from build123d import *

# Parameters (mm, degrees)
SKETCH1_W           = 53
SKETCH1_H           = 16
BOSS_EXTRUDE1_DEPTH = 18
SHELL1_T            = -0.5
SKETCH2_W           = 90
SKETCH2_H           = 20
SKETCH2_R           = 2.5
BOSS_EXTRUDE2_DEPTH = 0.5


with BuildPart() as part:
    # Sketch1 → Boss-Extrude1 (new body)
    with BuildSketch(Plane(origin=(0, 0, 0), x_dir=(0, 0, -1), z_dir=(1, 0, 0))):
        Rectangle(SKETCH1_W, SKETCH1_H)
    extrude(amount=BOSS_EXTRUDE1_DEPTH)

    # Shell1
    shell1_openings = [part.faces().sort_by_distance(p)[0] for p in [
        (18, 0, 0),
    ]]
    offset(amount=SHELL1_T, openings=shell1_openings, kind=Kind.INTERSECTION)

    # Sketch2 → Boss-Extrude2 (add)
    with BuildSketch(Plane(origin=(18, 0, 0), x_dir=(0, 0, -1), z_dir=(1, 0, 0))):
        Rectangle(SKETCH2_W, SKETCH2_H)
        with Locations((36.5, 0)):
            Circle(SKETCH2_R, mode=Mode.SUBTRACT)
        with Locations((-36.5, 0)):
            Circle(SKETCH2_R, mode=Mode.SUBTRACT)
        Polygon((-16, 3.5), (-15, 3.5), (-15, 5.5), (15, 5.5), (15, 3.5), (16, 3.5), (16, -3.5), (15, -3.5), (15, -5.5), (-15, -5.5), (-15, -3.5), (-16, -3.5), align=None, mode=Mode.SUBTRACT)
    extrude(amount=BOSS_EXTRUDE2_DEPTH)


solid = part.part
Can you work these out from the model? Positions are in its coordinate system, mm. A direction names the side the tool comes from. Round coordinates to 2 decimals unless told otherwise and drop trailing zeros. Write each loop counter-clockwise with the first axis right and the second up, starting at its lowest first coordinate (ties: lowest second). Pieces come first, ordered by that corner, then holes. Notation, with made-up numbers: (76.25, 15) -> (87.25, 15) arc R28 ccw to (87.25, 46) -> close; hole circle Ø4 at (-36, -12). An arc over 180 degrees is marked (long way). Use one line per item in the form item = value. Start each with the question number.
Q1. If I drill on probe 1 along Y at (x, z) = (15.75, -16.5); probe 2 along Z at (x, y) = (7.75, 1.5); probe 3 along X at (y, z) = (1.75, 18), over which ranges is the centre line in solid material (lowest first)? Write a range as [from, to].
Q2. Imagine slicing it at D-D (z = -13). Please give me the cut outline in (x, y).
Q3. We'd pull the mould along Y, two halves only. Please class faces 6 (the face through (9, 0, 26.5)), 7 (the face through (9, 8, 0)), 8 (the face through (9, -7.5, 0)): +Y half, -Y half, draft (parallel to the pull), parting line (faces both ways), or undercut.
Q4. Imagine slicing it at B-B (y = 0). Please give me the cut outline in (x, z).
Q5. Imagine slicing it at C-C (x = 9.5). Please give me the cut outline in (y, z), then the cut area to 3 significant figures.
Q6. I'm going to push flat-ended pins straight in: P1, Ø5.5, axis at x = 10, z = 7.5, coming from the +Y side; P2, Ø8, axis at x = 8, y = -3, coming from the -Z side; P3, Ø6.5, axis at y = 0, z = -36.5, coming from the -X side. Where does each tip first touch, or does it pass through?
Q7. Which directions (+Z, -Z, +X, -X, +Y, -Y) give clear straight access to the entire face, cutting with the end or side of a thin tool? Please do faces 1 (the face through (9, 0, -26.5)), 2 (the face through (0, 0, 0)), 3 (the face through (18, -7, 0)), 4 (the face through (18.5, 7, 1)), 5 (the face through (9, -8, 0)).
Q8. Imagine slicing it at A-A (z = 36.5). Please give me the cut outline in (x, y).
Worked out:
q1.probe_1 = [-8, -7.5], [7.5, 8]
q1.probe_2 = [-26.5, -26], [26, 26.5]
q1.probe_3 = [0, 0.5], [18, 18.5]
q2.outline = (0, -8) -> (18, -8) -> (18, -10) -> (18.5, -10) -> (18.5, -5.5) -> (18, -5.5) -> (18, -7.5) -> (0.5, -7.5) -> (0.5, 7.5) -> (18, 7.5) -> (18, 5.5) -> (18.5, 5.5) -> (18.5, 10) -> (18, 10) -> (18, 8) -> (0, 8) -> close
q3.face_6 = draft
q3.face_7 = +Y half
q3.face_8 = undercut
q4.outline = (0, -26.5) -> (18, -26.5) -> (18, -34) -> (18.5, -34) -> (18.5, -16) -> (18, -16) -> (18, -26) -> (0.5, -26) -> (0.5, 26) -> (18, 26) -> (18, 16) -> (18.5, 16) -> (18.5, 34) -> (18, 34) -> (18, 26.5) -> (0, 26.5) -> close; (18, -45) -> (18.5, -45) -> (18.5, -39) -> (18, -39) -> close; (18, 39) -> (18.5, 39) -> (18.5, 45) -> (18, 45) -> close
q5.outline = (-8, -26.5) -> (8, -26.5) -> (8, 26.5) -> (-8, 26.5) -> close; hole (-7.5, -26) -> (7.5, -26) -> (7.5, 26) -> (-7.5, 26) -> close
q5.area = 68.0 mm^2
q6.P1 = 8
q6.P2 = -26.5
q6.P3 = 18
q7.face_1 = -Z, -X, +Y, -Y
q7.face_2 = +Z, -Z, -X, +Y, -Y
q7.face_3 = none
q7.face_4 = +Z, -Z, +X, +Y, -Y
q7.face_5 = +Z, -Z, -X, -Y
q8.outline = (18, -10) -> (18.5, -10) -> (18.5, -2.5) -> (18, -2.5) -> close; (18, 2.5) -> (18.5, 2.5) -> (18.5, 10) -> (18, 10) -> close
